Read the model definition and answer for the solid it produces. Units are mm, in the model's axes. Face numbers are marked on the shaded views. A direction names the side the tool comes from. Coordinates: 2 decimals unless noted, no trailing zeros. Loops run counter-clockwise (first coordinate to the right, second up) from the corner with the lowest first, then second, coordinate; pieces in that order, holes last. Notation, with made-up numbers: (-30, -10.5) -> (-22, -10.5) arc R21 ccw to (-22, 17.5) -> close; hole circle Ø2 at (78, 27). An arc over 180 degrees is marked (long way). Answer as a JSON object with one key per item and string values. Group by question number.
1) Section D-D, the plane y = 11.25 is taken. Give the vertices of the cut face in (x, z), plus the area to 3 significant figures.
2) Which of the six approach directions +Z, -Z, +X, -X, +Y, -Y give full straight-line access (tool end or side, diameter ignored) to the marked faces 5 and 6?
3) Section B-B, the plane z = 1.9 is taken. Give the vertices of the cut face in (x, y) (3 decimals), plus the area to 3 significant figures.
4) Section A-A, the plane y = 4.75 is taken. Give the vertices of the cut face in (x, z), plus the area to 3 significant figures.
5) Section C-C, the plane x = 6.75 is taken. Give the vertices of the cut face in (y, z).
6) Consider probe 1 along X at (y, z) = (4.25, 1.6); probe 2 along X at (y, z) = (5.75, 2.8); probe 3 along Y at (x, z) = (9.5, 2.1). Determine where each line is inside the solid, lowest interval first. Write a range as [from, to].
7) Determine the mould class of the marked faces 1, 2, 3 and 4 for opening direction Y: released by +Y, released by -Y, zero draft, split by the parting line, or undercut.
8) Flat-ended cylindrical pins translate along their axes: P1, Ø1, axis at y = 4, z = 1, coming from the +X side; P2, Ø1.1, axis at y = 10.5, z = 2, coming from the +X side; P3, Ø1.1, axis at y = 10, z = 1.5, coming from the -X side; P4, Ø2, axis at x = 0, y = 11, coming from the -Z side. Find the tip coordinate at first contact, or state that the pin passes through.
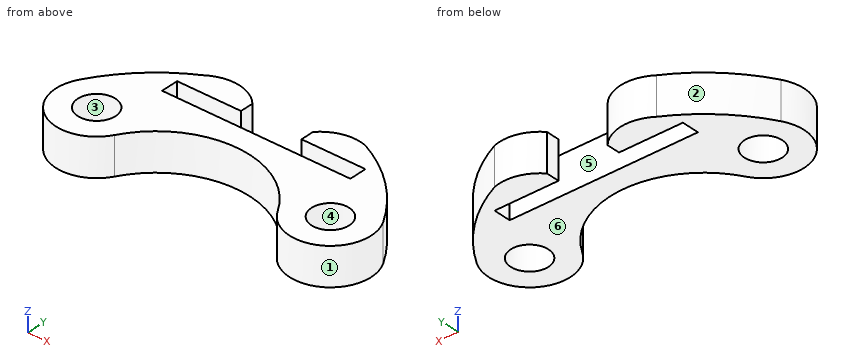
from build123d import *

# Parameters (mm, degrees)
ESQUISSE1_R        = 1.5
BOSS_EXTRU_2_DEPTH = 3


with BuildPart() as part:
    # Esquisse1 → Boss.-Extru.2 (new body)
    with BuildSketch(Plane.XY):
        with BuildLine():
            Line((-2.411034891, 11.820685714), (-2.411034891, 10.75))
            Line((-2.411034891, 10.75), (-7.5, 10.75))
            Line((-7.5, 10.75), (-7.5, 9.35))
            Line((-7.5, 9.35), (7.5, 9.35))
            Line((7.5, 9.35), (7.5, 10.75))
            Line((7.5, 10.75), (2.411034891, 10.75))
            Line((2.411034891, 10.75), (2.411034891, 11.820685714))
            ThreePointArc((2.411034891, 11.820685714), (3.975330286, 12.779130538), (5.80943088, 12.737759334))
            ThreePointArc((5.80943088, 12.737759334), (9.414650572, 10.36167721), (12.124355653, 7))
            ThreePointArc((12.124355653, 7), (10.934773091, 2.560417438), (6.495190528, 3.75))
            ThreePointArc((6.495190528, 3.75), (0, 7.5), (-6.495190528, 3.75))
            ThreePointArc((-6.495190528, 3.75), (-10.934773091, 2.560417438), (-12.124355653, 7))
            ThreePointArc((-12.124355653, 7), (-9.780131311, 10.017436376), (-6.707371512, 12.288660114))
            ThreePointArc((-6.707371512, 12.288660114), (-4.47014813, 12.872261577), (-2.411034891, 11.820685714))
        make_face()
        with Locations((9.309773091, 5.375)):
            Circle(ESQUISSE1_R, mode=Mode.SUBTRACT)
        with Locations((-9.309773091, 5.375)):
            Circle(ESQUISSE1_R, mode=Mode.SUBTRACT)
    extrude(amount=BOSS_EXTRU_2_DEPTH)


solid = part.part
Determined:
{
 "1": {"outline": "(-8.33, 0) -> (-2.41, 0) -> (-2.41, 3) -> (-8.33, 3) -> close; (2.41, 0) -> (8.33, 0) -> (8.33, 3) -> (2.41, 3) -> close", "area": "35.5 mm²"},
 "2": {"face 5": "+Z, -Z", "face 6": "-Z, +X, -X, +Y, -Y"},
 "3": {"outline": "(-12.124, 7) arc R3.25 ccw to (-6.495, 3.75) arc R7.5 cw to (6.495, 3.75) arc R3.25 ccw to (12.124, 7) arc R14 ccw to (5.809, 12.738) arc R3.25 ccw to (2.411, 11.821) -> (2.411, 10.75) -> (7.5, 10.75) -> (7.5, 9.35) -> (-7.5, 9.35) -> (-7.5, 10.75) -> (-2.411, 10.75) -> (-2.411, 11.821) arc R3.25 ccw to (-6.707, 12.289) arc R14 ccw to start; hole circle Ø3 at (-9.31, 5.375); hole circle Ø3 at (9.31, 5.375)", "area": "124 mm²"},
 "4": {"outline": "(-12.5, 0) -> (-10.67, 0) -> (-10.67, 3) -> (-12.5, 3) -> close; (-7.95, 0) -> (-5.8, 0) -> (-5.8, 3) -> (-7.95, 3) -> close; (5.8, 0) -> (7.95, 0) -> (7.95, 3) -> (5.8, 3) -> close; (10.67, 0) -> (12.5, 0) -> (12.5, 3) -> (10.67, 3) -> close", "area": "23.8 mm²"},
 "5": {"outline": "(3.37, 0) -> (9.35, 0) -> (9.35, 3) -> (3.37, 3) -> close; (10.75, 0) -> (12.27, 0) -> (12.27, 3) -> (10.75, 3) -> close"},
 "6": {"probe 1": "[-12.36, -10.3], [-8.32, -6.18], [6.18, 8.32], [10.3, 12.36]", "probe 2": "[-12.54, -10.76], [-7.86, -4.82], [4.82, 7.86], [10.76, 12.54]", "probe 3": "[2.13, 3.89], [6.86, 10.28]"},
 "7": {"face 1": "split by the parting line", "face 2": "released by +Y", "face 3": "undercut", "face 4": "undercut"},
 "8": {"P1": "x = 12.44", "P2": "x = 9.85", "P3": "x = -10.33", "P4": "through"}
}
